from build123d import *

# Parameters (mm, degrees)
KES_EKSTR_ZYON1_DEPTH = 457.345778602
IZIM3_R               = 14
KES_EKSTR_ZYON2_DEPTH = 40
KES_EKSTR_ZYON3_DEPTH = 40


with BuildPart() as part:
    # Çizim1 → Döndür1 (revolve)
    with BuildSketch(Plane(origin=(0, 0, 414.673045167), x_dir=(-1, 0, 0), z_dir=(0, 0, -1)), mode=Mode.PRIVATE) as d_nd_r1_sk:
        Polygon((-985.254127108, 38.3), (-985.254127108, 0), (-945.254127108, 0), (-945.254127108, 38.3), (-948.254127108, 38.3), (-951.695071737, 26.3), (-958.813182479, 26.3), (-962.254127108, 38.3), (-968.254127108, 38.3), (-971.695071737, 26.3), (-978.813182479, 26.3), (-982.254127108, 38.3), align=None)
    revolve(d_nd_r1_sk.sketch.rotate(Axis((985.254127108, 0, 414.673045167), (-1, 0, 0)), 270), axis=Axis((985.254127108, 0, 414.673045167), (-1, 0, 0)))

    # Çizim2 → Kes-Ekstrüzyon1 (cut, through all)
    with BuildSketch(Plane.ZY.offset(-945.254127108)):
        with BuildLine():
            Line((405.659166978, 3), (402.173045167, 3))
            Line((402.173045167, 3), (402.173045167, -3))
            Line((402.173045167, -3), (405.659166978, -3))
            ThreePointArc((405.659166978, -3), (424.173045167, 0), (405.659166978, 3))
        make_face()
    extrude(amount=-KES_EKSTR_ZYON1_DEPTH, mode=Mode.SUBTRACT)

    # Çizim3 → Kes-Ekstrüzyon2 (cut)
    with BuildSketch(Plane(origin=(985.254127108, 0, 0), x_dir=(0, 0, -1), z_dir=(1, 0, 0))):
        with Locations((-414.673045167, 0)):
            Circle(IZIM3_R)
    extrude(amount=-KES_EKSTR_ZYON2_DEPTH, mode=Mode.SUBTRACT)

    # Çizim4 → Kes-Ekstrüzyon3 (cut)
    with BuildSketch(Plane(origin=(985.254127108, 0, 0), x_dir=(0, 0, -1), z_dir=(1, 0, 0))):
        Polygon((-400.673045167, 4), (-400.673045167, 0), (-400.673045167, -4), (-397.173045167, -4), (-397.173045167, 4), align=None)
        with BuildLine():
            ThreePointArc((-401.256637302, 4), (-400.819711451, 2.02117415), (-400.673045167, 0))
            Line((-400.673045167, 0), (-400.673045167, 4))
            Line((-400.673045167, 4), (-401.256637302, 4))
        make_face()
        with BuildLine():
            Line((-400.673045167, -4), (-400.673045167, 0))
            ThreePointArc((-400.673045167, 0), (-400.819711451, -2.02117415), (-401.256637302, -4))
            Line((-401.256637302, -4), (-400.673045167, -4))
        make_face()
    extrude(amount=-KES_EKSTR_ZYON3_DEPTH, mode=Mode.SUBTRACT)


solid = part.part
Could you check a few things on this model? Use its own coordinates, in mm. A direction names the side the tool comes from. Coordinates: 2 decimals unless noted, no trailing zeros. Order: outer loops, then holes, each group sorted by start corner. A loop starts at its lowest first (then second) coordinate and runs counter-clockwise, first axis right, second up.
Q1. Please list where these lines run through material, in increasing order: L1, parallel to X at y = 33, z = 408; L2, parallel to X at y = -9, z = 386; L3, parallel to Z at x = 963.5, y = -9.
Q2. Thinking about a two-plate mould opening in Z: for faces 1 (the cylindrical face through (955.3, -10.07, 438.97)), 2 (the flat face through (966, -4, 399)), 3 (the flat face through (945.254, -16, 415)), which applies, released by +Z, released by -Z, zero draft, split by the parting line, or undercut?
Q3. Which directions (+Z, -Z, +X, -X, +Y, -Y) give clear straight access to the entire face, cutting with the end or side of a thin tool? Please do faces 4 (the flat face through (966, 0, 397.173)), 5 (the flat face through (985.254, 1, 431)), 6 (the conical face through (979.03, 1.19, 387.65)).
Q4. Will these pins go through, and if not, where does the flat tip stop? pin 1 (5 mm diameter, centred on x = 981, z = 435.5, fed in from -Y); pin 2 (10 mm diameter, centred on x = 971.5, y = -14, fed in from +Z); pin 3 (2 mm diameter, centred on x = 977.5, z = 396.5, fed in from -Y).
Q5. Suppose I cut it at D-D on z = 386. Give the number of separate pieces and of enclosed holes in the cut face, and give its area (3 significant figures).
Q6. Suppose I cut it at C-C on x = 975. Please give me the cut outline in (y, z).
Q7. Suppose I cut it at B-B on x = 966. Please give me the cut outline in (y, z), and give its area (3 significant figures).
Q8. Suppose I cut it at A-A on y = 0. Please give me the cut outline in (x, z), and give its area (3 significant figures).
Answer:
1. L1: x = 945.25 to 949.58, 960.93 to 969.58, 980.93 to 985.25
1. L2: x = 945.25 to 950.62, 959.89 to 970.62, 979.89 to 985.25
1. L3: z = 377.45 to 403.95, 425.4 to 451.9
2. face 1: split by the parting line
2. face 2: undercut
2. face 3: zero draft
3. face 4: +X, -X
3. face 5: +Z, -Z, +X, +Y, -Y
3. face 6: none
4. pin 1: stops at y = -33.44
4. pin 2: stops at z = 451.59
4. pin 3: stops at y = -19.92
5. separate pieces: 3
5. enclosed holes: 0
5. area: 972 mm2
6. outline: circle Ø52.6 at (0, 414.67); hole (-4, 397.17) - (4, 397.17) - (4, 401.26) arc R14 ccw (long way) to (-4, 401.26) - close
7. outline: circle Ø76.6 at (0, 414.67); hole (-4, 397.17) - (4, 397.17) - (4, 401.26) arc R14 ccw (long way) to (-4, 401.26) - close
7. area: 3,960 mm2
8. outline: (945.25, 376.37) - (948.25, 376.37) - (951.7, 388.37) - (958.81, 388.37) - (962.25, 376.37) - (968.25, 376.37) - (971.7, 388.37) - (978.81, 388.37) - (982.25, 376.37) - (985.25, 376.37) - (985.25, 397.17) - (945.25, 397.17) - close; (945.25, 428.67) - (985.25, 428.67) - (985.25, 452.97) - (982.25, 452.97) - (978.81, 440.97) - (971.7, 440.97) - (968.25, 452.97) - (962.25, 452.97) - (958.81, 440.97) - (951.7, 440.97) - (948.25, 452.97) - (945.25, 452.97) - close
8. area: 1,300 mm2
